```python
from build123d import *

# Parameters (mm, degrees)
EXTRUDE003_DEPTH  = 3.6
CYLINDER002_R     = 1.35
CYLINDER002_DEPTH = 3.4
EXTRUDE002_DEPTH  = 1.8
CYLINDER003_R     = 1.35
CYLINDER003_DEPTH = 3.4
EXTRUDE001_DEPTH  = 1.8
CYLINDER_R        = 1.35
CYLINDER_DEPTH    = 3.4
BOX_W             = 22
BOX_H             = 3.4
BOX_DEPTH         = 14.5
BOX001_W          = 12.7
BOX001_H          = 4.6
BOX001_DEPTH      = 3.4
EXTRUDE_DEPTH     = 3.4


with BuildPart() as extrude003:
    # Sketch003 → Extrude003 (new body)
    with BuildSketch(Plane(origin=(5.5, -1, 1.6), x_dir=(1, 0, 0), z_dir=(0, 0, 1))):
        Polygon((3, 0), (1.5, 2.598076), (-1.5, 2.598076), (-3, 0), (-1.5, -2.598076), (1.5, -2.598076), align=None)
    extrude(amount=EXTRUDE003_DEPTH)


with BuildPart() as hole03:
    # Cylinder002 → Cylinder002 (new body)
    with BuildSketch(Plane(origin=(5.5, -1, 0), x_dir=(0, 1, 0), z_dir=(0, 0, 1))):
        Circle(CYLINDER002_R)
    extrude(amount=CYLINDER002_DEPTH)

    # Fusion002: union Extrude003
    add(extrude003.part)


with BuildPart() as extrude002:
    # Sketch002 → Extrude002 (new body)
    with BuildSketch(Plane(origin=(16.5, 1.8, 9), x_dir=(1, 0, 0), z_dir=(0, -1, 0))):
        Polygon((3, 0), (1.5, 2.598076), (-1.5, 2.598076), (-3, 0), (-1.5, -2.598076), (1.5, -2.598076), align=None)
    extrude(amount=EXTRUDE002_DEPTH)


with BuildPart() as hole02:
    # Cylinder003 → Cylinder003 (new body)
    with BuildSketch(Plane(origin=(16.5, 3.4, 9), x_dir=(1, 0, 0), z_dir=(0, -1, 0))):
        Circle(CYLINDER003_R)
    extrude(amount=CYLINDER003_DEPTH)

    # Fusion001: union Extrude002
    add(extrude002.part)


with BuildPart() as extrude001:
    # Sketch001 → Extrude001 (new body)
    with BuildSketch(Plane(origin=(5.5, 1.8, 9), x_dir=(1, 0, 0), z_dir=(0, -1, 0))):
        Polygon((3, 0), (1.5, 2.598076), (-1.5, 2.598076), (-3, 0), (-1.5, -2.598076), (1.5, -2.598076), align=None)
    extrude(amount=EXTRUDE001_DEPTH)


with BuildPart() as hole01:
    # Cylinder → Cylinder (new body)
    with BuildSketch(Plane(origin=(5.5, 3.4, 9), x_dir=(1, 0, 0), z_dir=(0, -1, 0))):
        Circle(CYLINDER_R)
    extrude(amount=CYLINDER_DEPTH)

    # Fusion: union Extrude001
    add(extrude001.part)


with BuildPart() as cut001:
    # Box → Box (new body)
    with BuildSketch(Plane.XY):
        with Locations((11, 1.7)):
            Rectangle(BOX_W, BOX_H)
    extrude(amount=BOX_DEPTH)

    # Cut: cut Hole01
    add(hole01.part, mode=Mode.SUBTRACT)

    # Cut001: cut Hole02
    add(hole02.part, mode=Mode.SUBTRACT)


with BuildPart() as cut002:
    # Box001 → Box001 (new body)
    with BuildSketch(Plane(origin=(0, -4.6, 0), x_dir=(1, 0, 0), z_dir=(0, 0, 1))):
        with Locations((6.35, 2.3)):
            Rectangle(BOX001_W, BOX001_H)
    extrude(amount=BOX001_DEPTH)

    # Fusion003: union Cut001
    add(cut001.part)

    # Cut002: cut Hole03
    add(hole03.part, mode=Mode.SUBTRACT)


with BuildPart() as left_hand_bracket:
    # Sketch → Extrude (new body)
    with BuildSketch(Plane(origin=(0, 0, 3.4), x_dir=(0, 1, 0), z_dir=(1, 0, 0))):
        Polygon((0, 11.1), (0, 0), (-4.6, 0), align=None)
    extrude(amount=EXTRUDE_DEPTH)


with BuildPart() as left_hand_bracket_1:
    # Extrude placement: moved
    add(left_hand_bracket.part.moved(Location((9.3, 0, 0))))

    # Fusion004: union Cut002
    add(cut002.part)


solid = left_hand_bracket_1.part
```
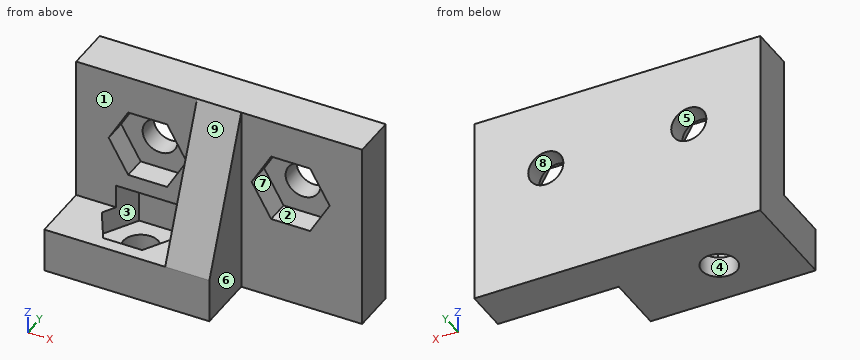
Design review of the part built by this model. Coordinates are the model's own, in mm. Face numbers are marked on the shaded views. A direction names the side the tool comes from. Coordinates: 2 decimals unless noted, no trailing zeros. Write each loop counter-clockwise with the first axis right and the second up, starting at its lowest first coordinate (ties: lowest second). Pieces come first, ordered by that corner, then holes.
1) Add section B-B (x = 4.5). Write out the cut boundary in (y, z), plus the area to 3 significant figures.
2) Machinability: for the marked faces 1, 2, 3, 4 and 5, which of the approach directions +Z, -Z, +X, -X, +Y, -Y give a long, thin tool a straight path to every point of the face, cutting with its end or side? Answer none if there is none.
3) Insertion check: pin 1 (5.5 mm diameter, centred on x = 5, z = 8, fed in from -Y); pin 2 (3.5 mm diameter, centred on x = 16.5, z = 9, fed in from -Y). Each pin has a flat end and moves straight along its axis. Give the tip position at first contact, or say it passes through.
4) To check wall thickness, follow L1, parallel to X at y = 2.45, z = 9; L2, parallel to Y at x = 5.5, z = 0.9; L3, parallel to Z at x = 15.5, y = 0.25. State the ranges of each line that lie inside material, in increasing order.
5) Add section D-D (x = 16.5). Write out the cut boundary in (y, z).
6) Mouldability with a two-part tool opening along X and no side actions: class the marked faces 6, 7, 8 and 9 as +X half, -X half, draft (parallel to the pull), parting line (faces both ways), or undercut.
7) Add section A-A (z = 2.25). Write out the cut boundary in (x, y), plus the area to 3 significant figures.
8) Add section C-C (y = 3). Write out the cut boundary in (x, z), plus the area to 3 significant figures.
Check result:
1. outline: (-4.6, 0) - (-1.91, 0) - (-1.91, 1.6) - (-3.6, 1.6) - (-3.6, 3.4) - (-4.6, 3.4) - close; (-0.09, 0) - (3.4, 0) - (3.4, 8.09) - (1.8, 8.09) - (1.8, 6.4) - (0, 6.4) - (0, 5.2) - (1.6, 5.2) - (1.6, 1.6) - (-0.09, 1.6) - close; (0, 11.6) - (1.8, 11.6) - (1.8, 9.91) - (3.4, 9.91) - (3.4, 14.5) - (0, 14.5) - close
1. area: 37.6 mm2
2. face 1: +Z, -X, -Y
2. face 2: -Y
2. face 3: none
2. face 4: -Z
2. face 5: +Y, -Y
3. pin 1: stops at y = 0
3. pin 2: stops at y = 1.8
4. L1: x = 0 to 4.15, 6.85 to 15.15, 17.85 to 22
4. L2: y = -4.6 to -2.35, 0.35 to 3.4
4. L3: z = 0 to 6.4, 11.6 to 14.5
5. outline: (0, 0) - (3.4, 0) - (3.4, 7.65) - (1.8, 7.65) - (1.8, 6.4) - (0, 6.4) - close; (0, 11.6) - (1.8, 11.6) - (1.8, 10.35) - (3.4, 10.35) - (3.4, 14.5) - (0, 14.5) - close
6. face 6: +X half
6. face 7: undercut
6. face 8: undercut
6. face 9: draft
7. outline: (0, -4.6) - (12.7, -4.6) - (12.7, 0) - (22, 0) - (22, 3.4) - (0, 3.4) - close; hole (2.5, -1) - (4, -3.6) - (7, -3.6) - (8.5, -1) - (7, 1.6) - (4, 1.6) - close
7. area: 110 mm2
8. outline: (0, 0) - (22, 0) - (22, 14.5) - (0, 14.5) - close; hole circle Ø2.7 at (5.5, 9); hole circle Ø2.7 at (16.5, 9)
8. area: 308 mm2
